Verification items for this drawing (mm, ordinates from the low corner). Coordinates: 2 decimals unless noted, no trailing zeros. Order: outer loops, then holes, each group sorted by start corner. A loop starts at its lowest first (then second) coordinate and runs counter-clockwise, first axis right, second up. Notation, with made-up numbers: (32, 56.25) -> (46, 56.25) arc R14 cw to (46, 76.25) -> close; hole circle Ø1 at (13, -32.5). An arc over 180 degrees is marked (long way). Write each question's results on one line, items separated by ' | '. Start each with the question number.
(1) Cross-section at A-A on x = 37.5. Enter the section's corners in (y, z).
(2) Go/stop test with flat-tipped pins: pin 1 (1.5 mm diameter, centred on y = 22.5, z = 20.5, fed in from -X); pin 2 (2 mm diameter, centred on x = 35, y = 35.5, fed in from +Z); pin 3 (2 mm diameter, centred on x = 56.5, y = 23.5, fed in from +Z). Record where each tip stops, or that it passes through.
(3) Cross-section at D-D on z = 17. Enter the section's corners in (x, y).
(4) Draft check along X on the marked faces 1, 2, 3 and 4. Enter one of: +X half, -X half, draft (parallel to the pull), parting line (faces both ways), or undercut.
(5) Cross-section at C-C on z = 30.5. Enter the section's corners in (x, y).
(6) Thickness scan on probe 1 along Y at (x, z) = (32.5, 26); probe 2 along Y at (x, z) = (39, 30.5) (1 decimal); probe 3 along Z at (x, y) = (41, 56). Record the ranges inside material, lowest first. Write a range as [from, to].
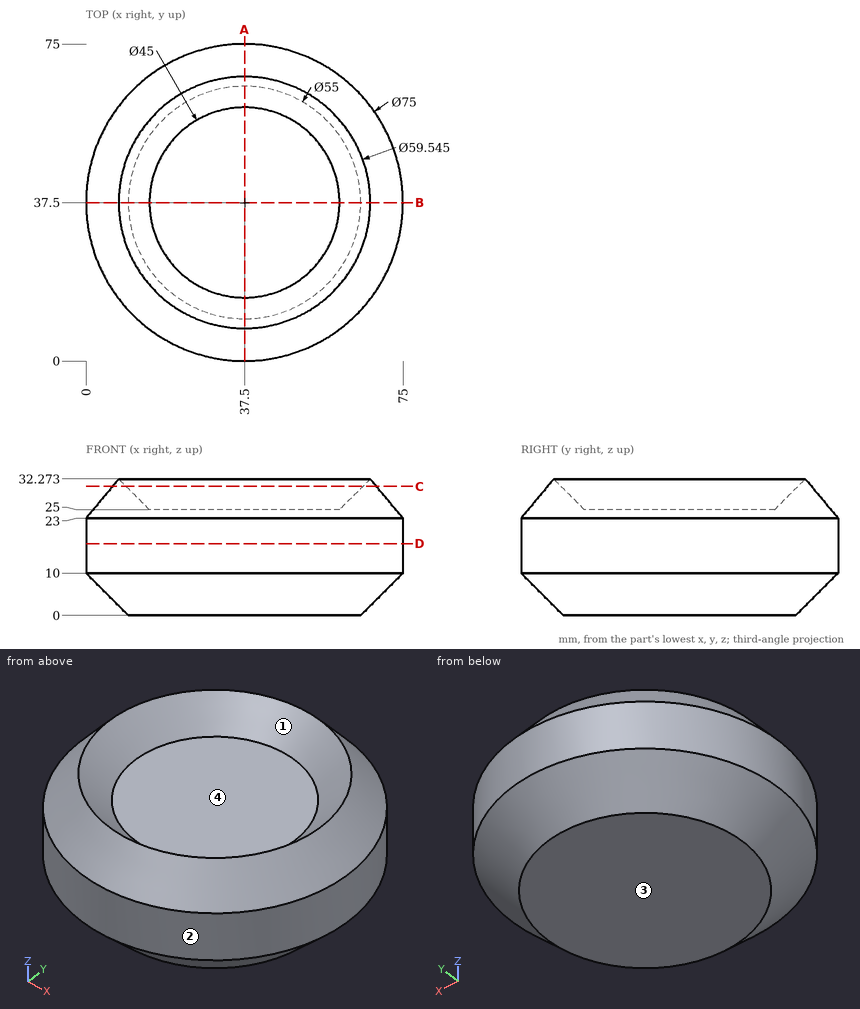
Results are:
1) outline: (0, 10) -> (10, 0) -> (65, 0) -> (75, 10) -> (75, 23) -> (67.27, 32.27) -> (60, 25) -> (15, 25) -> (7.73, 32.27) -> (0, 23) -> close
2) pin 1: stops at x = 2.81 | pin 2: stops at z = 25 | pin 3: stops at z = 27.1
3) outline: circle Ø75 at (37.5, 37.5)
4) face 1: undercut | face 2: parting line | face 3: draft | face 4: undercut
5) outline: circle Ø62.5 at (37.5, 37.5); hole circle Ø56 at (37.5, 37.5)
6) probe 1: y = [2.86, 14.54], [60.46, 72.14] | probe 2: y = [6.3, 9.5], [65.5, 68.7] | probe 3: z = [0, 25]
